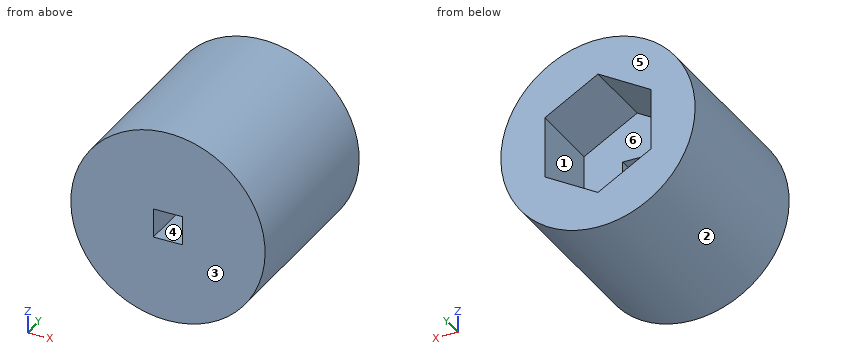
from build123d import *

# Parameters (mm, degrees)
SKETCH1_R           = 10.16
BOSS_EXTRUDE1_DEPTH = 19.05
CUT_EXTRUDE1_DEPTH  = 7.9375
SKETCH2_W           = 3.048
SKETCH2_H           = 3.048
CUT_EXTRUDE2_DEPTH  = 11.1125


with BuildPart() as part:
    # Sketch1 → Boss-Extrude1 (new body)
    with BuildSketch(Plane(origin=(0, 0, 0), x_dir=(1, 0, 0), z_dir=(0, 1, 0))):
        with Locations(Location((0, 0, 0), (0, 0, 90))):
            Circle(SKETCH1_R)
    extrude(amount=BOSS_EXTRUDE1_DEPTH)

    # Sketch3 → Cut-Extrude1 (cut)
    with BuildSketch(Plane(origin=(0, 19.05, 0), x_dir=(1, 0, 0), z_dir=(0, 1, 0))):
        Polygon((0, -6.415804866), (5.55625, -3.207902433), (5.55625, 3.207902433), (0, 6.415804866), (-5.55625, 3.207902433), (-5.55625, -3.207902433), align=None)
    extrude(amount=-CUT_EXTRUDE1_DEPTH, mode=Mode.SUBTRACT)

    # Sketch2 → Cut-Extrude2 (cut)
    with BuildSketch(Plane(origin=(0, 0, 0), x_dir=(-1, 0, 0), z_dir=(0, -1, 0))):
        Rectangle(SKETCH2_W, SKETCH2_H)
    extrude(amount=-CUT_EXTRUDE2_DEPTH, mode=Mode.SUBTRACT)


solid = part.part
Input: part model. Units: mm. Frame: model coordinates. Face numbers are marked on the shaded views. A direction names the side the tool comes from. Give positions to 0.01 mm unless a question says otherwise; leave off trailing zeros. Loops run counter-clockwise (first coordinate to the right, second up) from the corner with the lowest first, then second, coordinate; pieces in that order, holes last. Notation, with made-up numbers: M 18,19 L 48,19 A26 ccw 48,41 Z; hole C 21,12 d3. An arc over 180 degrees is marked long. Use CSV: the item, a comma, the result in double quotes.
(1) Pin query (flat end, axial travel): P1, Ø1.5, axis at x = 2.5, z = -2.5, coming from the +Y side; P2, Ø10, axis at y = 17, z = 5.5, coming from the +X side; P3, Ø2, axis at y = 10.5, z = -4.5, coming from the +X side. Return the tip coordinate at first contact, or that it passes through.
Outcome:
P1,"stops at y = 11.11"
P2,"stops at x = 10.15"
P3,"stops at x = 9.54"
(2) Pull-direction query (Z, two-part tool) for the marked faces 1, 2 and 3; classes: pulls with the +Z half, pulls with the -Z half, needs draft (parallel to the pull), parting line crosses it, or undercut.
Outcome:
face 1,"undercut"
face 2,"parting line crosses it"
face 3,"needs draft"
(3) Section C-C, the plane x = 2.75. Return loops of the section in (y, z), plus the area to 3 significant figures.
Outcome:
outline,"M 0,-9.78 L 19.05,-9.78 L 19.05,-4.83 L 11.11,-4.83 L 11.11,4.83 L 19.05,4.83 L 19.05,9.78 L 0,9.78 Z"
area,"296 mm²"
(4) Set-up query: the marked faces 4, 5 and 6. Return all of +Z, -Z, +X, -X, +Y, -Y with unobstructed straight access to the full face (end or side cutting, diameter ignored); none if empty.
Outcome:
face 4,"+Y, -Y"
face 5,"+Z, -Z, +X, -X, +Y"
face 6,"+Y"
(5) Section A-A, the plane z = 0. Return loops of the section in (x, y).
Outcome:
outline,"M -10.16,0 L -1.52,0 L -1.52,11.11 L -5.56,11.11 L -5.56,19.05 L -10.16,19.05 Z; M 1.52,0 L 10.16,0 L 10.16,19.05 L 5.56,19.05 L 5.56,11.11 L 1.52,11.11 Z"
(6) Section B-B, the plane y = 14.75. Return loops of the section in (x, z), plus the area to 3 significant figures.
Outcome:
outline,"C 0,0 d20.32; hole M -5.56,-3.21 L 0,-6.42 L 5.56,-3.21 L 5.56,3.21 L 0,6.42 L -5.56,3.21 Z"
area,"217 mm²"
(7) Material intervals for L1, parallel to X at y = 4.75, z = 0.25; L2, parallel to Y at x = 3, z = 1.75; L3, parallel to X at y = 8, z = -8.5, sorted ascending. Write a range as [from, to].
Outcome:
L1,"x = [-10.16, -1.52], [1.52, 10.16]"
L2,"y = [0, 11.11]"
L3,"x = [-5.57, 5.57]"
(8) Section D-D, the plane z = 4.25. Return loops of the section in (x, y).
Outcome:
outline,"M -9.23,0 L 9.23,0 L 9.23,19.05 L 3.75,19.05 L 3.75,11.11 L -3.75,11.11 L -3.75,19.05 L -9.23,19.05 Z"
